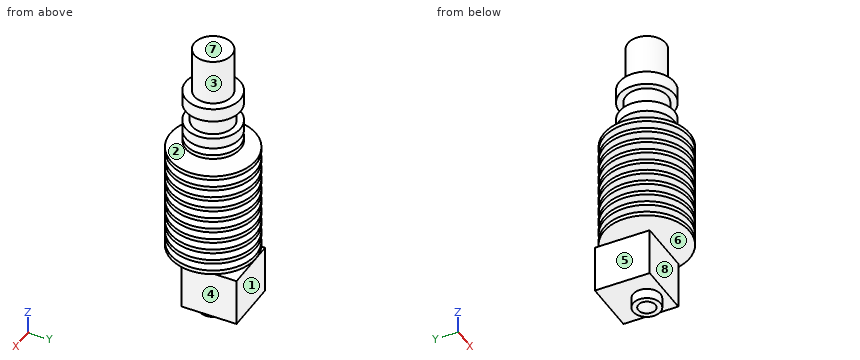
```python
from build123d import *

# Parameters (mm, degrees)
F2_W     = 16
F2_H     = 16
F3_DEPTH = 14


with BuildPart() as f1:
    # F0 (on Front) → F1 (revolve)
    with BuildSketch(Plane.XZ):
        Polygon((3, 0), (12.5, 0), (12.5, 1.2), (4.5, 1.2), (4.5, 3.422222), (12.5, 3.422222), (12.5, 4.622222), (4.5, 4.622222), (4.5, 6.844444), (12.5, 6.844444), (12.5, 8.044444), (4.5, 8.044444), (4.5, 10.266667), (12.5, 10.266667), (12.5, 11.466667), (4.5, 11.466667), (4.5, 13.688889), (12.5, 13.688889), (12.5, 14.888889), (4.5, 14.888889), (4.5, 17.111111), (12.5, 17.111111), (12.5, 18.311111), (4.5, 18.311111), (4.5, 20.533333), (12.5, 20.533333), (12.5, 21.733333), (4.5, 21.733333), (4.5, 23.955556), (12.5, 23.955556), (12.5, 25.155556), (4.5, 25.155556), (4.5, 27.377778), (12.5, 27.377778), (12.5, 28.577778), (4.5, 28.577778), (4.5, 30.8), (12.5, 30.8), (12.5, 32), (4.5, 32), (4.5, 34.222222), (8, 34.222222), (8, 35.422222), (4.5, 35.422222), (4.5, 37.644444), (8, 37.644444), (8, 40.844444), (6.1, 40.844444), (6.1, 46.444444), (8, 46.444444), (8, 50.444444), (5.5, 50.444444), (5.5, 64), (0, 64), (0, -2.5), (3, -2.5), align=None)
    revolve(axis=Axis((0, 0, 40.34683), (0, 0, -1)))

    # F2 (on face) → F3 (join)
    with BuildSketch(Plane(origin=(0, 0, -2.5), x_dir=(1, 0, 0), z_dir=(0, 0, -1))):
        with Locations((0, -3)):
            Rectangle(F2_W, F2_H)
    extrude(amount=F3_DEPTH)

    # F4 (on Front) → F5 (revolve)
    with BuildSketch(Plane.XZ):
        Polygon((0, -16.5), (0, -22.5), (2.5, -20.5), (4, -20.5), (4, -17.5), (2.5, -17.5), (2.5, -16.5), align=None)
    revolve(axis=Axis((0, 0, -19.509592), (0, 0, -1)))


solid = f1.part
```
Source: CAD feature listing. Evaluate the final solid. Frame: model axes, mm. Face numbers are marked on the shaded views. A direction names the side the tool comes from. Round coordinates to 2 decimals unless told otherwise and drop trailing zeros. Loops run counter-clockwise (first coordinate to the right, second up) from the corner with the lowest first, then second, coordinate; pieces in that order, holes last.
(1) Material intervals for probe 1 along Z at (x, y) = (-3, 2.5); probe 2 along Z at (x, y) = (1.25, -2.25); probe 3 along Z at (x, y) = (-3.75, 2), sorted ascending.
From the geometry:
probe 1: z = -20.5 to -17.5, -16.5 to -2.5, 0 to 64
probe 2: z = -20.5 to -17.5, -16.5 to 64
probe 3: z = -16.5 to -2.5, 0 to 64
(2) Pull-direction query (Z, two-part tool) for the marked faces 6, 7 and 8; classes: +Z half, -Z half, draft (parallel to the pull), parting line (faces both ways), or undercut.
From the geometry:
face 6: undercut
face 7: +Z half
face 8: draft
(3) Access query for the marked faces 1, 2, 3, 4 and 5. Directions: +Z, -Z, +X, -X, +Y, -Y. A direction counts if a zero-diameter tool reaches every point of the face in a straight line with its end or side. Return the directions, or none.
From the geometry:
face 1: -Z, +X, -X, +Y
face 2: none
face 3: +Z
face 4: -Z, +X, +Y, -Y
face 5: -Z, -X, +Y, -Y
(4) Section query A-A (z = -12.5). Output: boundary loops of the cut face in (x, y), and give its area (3 significant figures).
From the geometry:
outline: (-8, -5) - (8, -5) - (8, 11) - (-8, 11) - close
area: 256 mm2
(5) Contact query for flat-ended pins moving along their axis: pin 1 Ø7.5 at (x, y) = (0.5, 4) entering from -Z; pin 2 Ø10 at (y, z) = (6, 20) entering from -X; pin 3 Ø13 at (x, y) = (0.5, -3.5) entering from -Z; pin 4 Ø1.5 at (x, z) = (-10, 4) entering from -Y. Output: stop coordinate, or through.
From the geometry:
pin 1: stops at z = -22.28
pin 2: stops at x = -12.46
pin 3: stops at z = -22.5
pin 4: stops at y = -8.41
(6) Section query B-B (z = 5.5). Output: boundary loops of the cut face in (x, y), and give its area (3 significant figures).
From the geometry:
outline: circle Ø9 at (0, 0)
area: 63.6 mm2
